Verification items for the finished model (mm, model axes). A direction names the side the tool comes from. Coordinates: 2 decimals unless noted, no trailing zeros. Loops run counter-clockwise (first coordinate to the right, second up) from the corner with the lowest first, then second, coordinate; pieces in that order, holes last.
Q1. Go/stop test with flat-tipped pins: P1, Ø3.5, axis at x = -0.5, y = -1.5, coming from the -Z side; P2, Ø1.6, axis at y = -1, z = 4.5, coming from the +X side (3 decimals); P3, Ø1.1, axis at y = 3, z = 3.5, coming from the +X side. Record where each tip stops, or that it passes through.
Q2. Material ranges on probe 1 along Y at (x, z) = (-4.5, 2.25); probe 2 along Z at (x, y) = (-4.5, 5); probe 3 along Y at (x, z) = (-1.5, 1.75), recorded low to high.
Q3. Sectioned sample at C-C (z = -0.5). Enter the section's corners in (x, y).
Q4. Sectioned sample at A-A (x = 6). Enter the section's corners in (y, z).
Q5. Sectioned sample at B-B (y = 0.75). Enter the section's corners in (x, z) (3 decimals).
Q6. Mould release check, pull along Z, two halves, no side actions. Record for faces 4 (the face through (0, 7.62, 3)), 5 (the face through (24.79, 0.1, -0.5)), 6 (the face through (25.5, -0.1, 3.2)): +Z half, -Z half, draft (parallel to the pull), parting line (faces both ways), or undercut.
Q7. Access from +Z, -Z, +X, -X, +Y, -Y to the whole of each face (thin tool, end or side, straight path). Record for faces 1 (the face through (-24.765, 0, 2)), 2 (the face through (14.79, 0, 3)), 3 (the face through (24, 0, -1.1)).
Q8. Sectioned sample at D-D (x = -18). Enter the section's corners in (y, z).
```python
from build123d import *

# Parameters (mm, degrees)
SKETCH_W         = 52
SKETCH_H         = 15.24
PAD_DEPTH        = 5.2
CHAMFER_SIZE2    = 1
CHAMFER_SIZE     = 4
CHAMFER001_SIZE2 = 4
CHAMFER001_SIZE  = 1
SKETCH001_W      = 49.53
SKETCH001_H      = 12.24
POCKET_DEPTH     = 3.7
SKETCH002_W      = 1.21
SKETCH002_H      = 11.076
PAD001_DEPTH     = 2.5
SKETCH003_W      = 11.076
SKETCH003_H      = 1.4
PAD002_DEPTH     = 1.5
CHAMFER002_SIZE  = 1
SKETCH004_W      = 11.076
SKETCH004_H      = 1.4
PAD003_DEPTH     = 1.5
CHAMFER003_SIZE  = 1
SKETCH005_W      = 24.38
SKETCH005_H      = 7.58
POCKET001_DEPTH  = 1.5
SKETCH006_W      = 15
SKETCH006_H      = 1.5
PAD004_DEPTH     = 3.06
SKETCH007_W      = 1.5
SKETCH007_H      = 13
PAD005_DEPTH     = 1
SKETCH008_W      = 15
SKETCH008_H      = 1.5
PAD006_DEPTH     = 1.5
CHAMFER004_SIZE  = 1
SKETCH009_W      = 15
SKETCH009_H      = 1.5
PAD007_DEPTH     = 1.5
CHAMFER005_SIZE  = 1
SKETCH010_W      = 49.53
SKETCH010_H      = 15.24
POCKET002_DEPTH  = 1


with BuildPart() as part:
    # Sketch → Pad (new body)
    with BuildSketch(Plane.XY):
        Rectangle(SKETCH_W, SKETCH_H)
    extrude(amount=PAD_DEPTH)

    # Chamfer
    chamfer_edges = [part.edges().sort_by_distance(p)[0] for p in [
        (26, 0, 5.2),
    ]]
    chamfer_side = part.faces().sort_by_distance((26, 0, 2.6))[0]
    chamfer(chamfer_edges, length=CHAMFER_SIZE, length2=CHAMFER_SIZE2, reference=chamfer_side)

    # Chamfer001
    chamfer001_edges = [part.edges().sort_by_distance(p)[0] for p in [
        (-26, 0, 5.2),
    ]]
    chamfer001_side = part.faces().sort_by_distance((-0.5, 0, 5.2))[0]
    chamfer(chamfer001_edges, length=CHAMFER001_SIZE, length2=CHAMFER001_SIZE2, reference=chamfer001_side)

    # Sketch001 (on Face7 of Chamfer001) → Pocket (cut)
    with BuildSketch(Plane(origin=(0, 0, 0), x_dir=(1, 0, 0), z_dir=(0, 0, -1))):
        Rectangle(SKETCH001_W, SKETCH001_H)
    extrude(amount=-POCKET_DEPTH, mode=Mode.SUBTRACT)

    # Sketch002 (on Face7 of Pocket) → Pad001 (join)
    with BuildSketch(Plane(origin=(0, 0, 0), x_dir=(1, 0, 0), z_dir=(0, 0, -1))):
        with Locations((-25.395, 0)):
            Rectangle(SKETCH002_W, SKETCH002_H)
        with Locations((25.395, 0)):
            Rectangle(SKETCH002_W, SKETCH002_H)
    extrude(amount=PAD001_DEPTH)

    # Sketch003 (on Face15 of Pad001) → Pad002 (join)
    with BuildSketch(Plane.YZ.offset(-24.79)):
        with Locations((0, -1.8)):
            Rectangle(SKETCH003_W, SKETCH003_H)
    extrude(amount=PAD002_DEPTH)

    # Chamfer002
    chamfer002_edges = [part.edges().sort_by_distance(p)[0] for p in [
        (-23.29, 0, -2.5),
    ]]
    chamfer(chamfer002_edges, length=CHAMFER002_SIZE)

    # Sketch004 (on Face17 of Chamfer002) → Pad003 (join)
    with BuildSketch(Plane(origin=(24.79, 0, 0), x_dir=(0, -1, 0), z_dir=(-1, 0, 0))):
        with Locations((0, -1.8)):
            Rectangle(SKETCH004_W, SKETCH004_H)
    extrude(amount=PAD003_DEPTH)

    # Chamfer003
    chamfer003_edges = [part.edges().sort_by_distance(p)[0] for p in [
        (23.29, 0, -2.5),
    ]]
    chamfer(chamfer003_edges, length=CHAMFER003_SIZE)

    # Sketch005 (on Face25 of Chamfer003) → Pocket001 (cut)
    with BuildSketch(Plane.XY.offset(5.2)):
        with Locations((0, 0.8)):
            Rectangle(SKETCH005_W, SKETCH005_H)
    extrude(amount=-POCKET001_DEPTH, mode=Mode.SUBTRACT)

    # Sketch006 (on Face32 of Pocket001) → Pad004 (join)
    with BuildSketch(Plane(origin=(0, 0, 3.7), x_dir=(1, 0, 0), z_dir=(0, 0, -1))):
        with Locations((0, 6.66)):
            Rectangle(SKETCH006_W, SKETCH006_H)
        with Locations((0, -6.54)):
            Rectangle(SKETCH006_W, SKETCH006_H)
    extrude(amount=PAD004_DEPTH)

    # Sketch007 (on Face32 of Pad004) → Pad005 (join)
    with BuildSketch(Plane(origin=(0, 0, 3.7), x_dir=(1, 0, 0), z_dir=(0, 0, -1))):
        with Locations((14.04, 0)):
            Rectangle(SKETCH007_W, SKETCH007_H)
    extrude(amount=PAD005_DEPTH)

    # Sketch008 (on Face51 of Pad005) → Pad006 (join)
    with BuildSketch(Plane(origin=(0, -5.91, 0), x_dir=(-1, 0, 0), z_dir=(0, 1, 0))):
        with Locations((0, 1.39)):
            Rectangle(SKETCH008_W, SKETCH008_H)
    extrude(amount=PAD006_DEPTH)

    # Chamfer004
    chamfer004_edges = [part.edges().sort_by_distance(p)[0] for p in [
        (0, -4.41, 0.64),
    ]]
    chamfer(chamfer004_edges, length=CHAMFER004_SIZE)

    # Sketch009 (on Face15 of Chamfer004) → Pad007 (join)
    with BuildSketch(Plane.XZ.offset(-5.79)):
        with Locations((0, 1.39)):
            Rectangle(SKETCH009_W, SKETCH009_H)
    extrude(amount=PAD007_DEPTH)

    # Chamfer005
    chamfer005_edges = [part.edges().sort_by_distance(p)[0] for p in [
        (0, 4.29, 0.64),
    ]]
    chamfer(chamfer005_edges, length=CHAMFER005_SIZE)

    # Sketch010 → Pocket002 (cut)
    with BuildSketch(Plane.XY):
        Rectangle(SKETCH010_W, SKETCH010_H)
    extrude(amount=POCKET002_DEPTH, mode=Mode.SUBTRACT)


solid = part.part
```
Geometry check:
1. P1: stops at z = 3.7
1. P2: stops at x = 25.375
1. P3: stops at x = 25.56
2. probe 1: y = -7.62 to -5.91, 5.79 to 7.62
2. probe 2: z = 1 to 2.14, 3.7 to 5.2
2. probe 3: y = -7.62 to -4.41, 4.29 to 7.62
3. outline: (-26, -5.54) - (-24.79, -5.54) - (-24.79, 5.54) - (-26, 5.54) - close; (24.79, -5.54) - (26, -5.54) - (26, 5.54) - (24.79, 5.54) - close
4. outline: (-7.62, 1) - (-5.05, 1) - (-4.41, 1.64) - (-4.41, 2.14) - (-5.91, 2.14) - (-5.91, 3.7) - (-2.99, 3.7) - (-2.99, 5.2) - (-7.62, 5.2) - close; (4.29, 1.64) - (4.93, 1) - (7.62, 1) - (7.62, 5.2) - (4.59, 5.2) - (4.59, 3.7) - (5.79, 3.7) - (5.79, 2.14) - (4.29, 2.14) - close
5. outline: (-26, -2.5) - (-24.29, -2.5) - (-23.29, -1.5) - (-23.29, -1.1) - (-24.79, -1.1) - (-24.79, 0) - (-24.765, 0) - (-24.765, 3.7) - (-12.19, 3.7) - (-12.19, 5.2) - (-25, 5.2) - (-26, 1.2) - close; (12.19, 3.7) - (13.29, 3.7) - (13.29, 2.7) - (14.79, 2.7) - (14.79, 3.7) - (24.765, 3.7) - (24.765, 0) - (24.79, 0) - (24.79, -1.1) - (23.29, -1.1) - (23.29, -1.5) - (24.29, -2.5) - (26, -2.5) - (26, 1.2) - (25, 5.2) - (12.19, 5.2) - close
6. face 4: draft
6. face 5: undercut
6. face 6: +Z half
7. face 1: none
7. face 2: -Z
7. face 3: +Y, -Y
8. outline: (-7.62, 1) - (-6.12, 1) - (-6.12, 3.7) - (6.12, 3.7) - (6.12, 1) - (7.62, 1) - (7.62, 5.2) - (-7.62, 5.2) - close
